from build123d import *

# Parameters (mm, degrees)
SKETCH_1_R      = 1.4
EXTRUDE_1_DEPTH = 7


with BuildPart() as part:
    # 草图1 → 凸台-拉伸1 (new body)
    with BuildSketch(Plane.XY):
        with BuildLine():
            Line((-42.056135012, 57.617545139), (22.139601015, 67.811046791))
            ThreePointArc((22.139601015, 67.811046791), (31.867424404, 60.749216142), (24.805593755, 51.021392753))
            Line((24.805593755, 51.021392753), (-39.390142272, 40.827891101))
            ThreePointArc((-39.390142272, 40.827891101), (-40.473181997, 40.726394111), (-41.560315394, 40.764045938))
            ThreePointArc((-41.560315394, 40.764045938), (-42.147831339, 41.031589211), (-42.44945072, 41.60236074))
            Line((-42.44945072, 41.60236074), (-44.725061471, 55.933501507))
            ThreePointArc((-44.725061471, 55.933501507), (-44.615083087, 56.569629752), (-44.139340913, 57.006005475))
            ThreePointArc((-44.139340913, 57.006005475), (-43.117343546, 57.378561601), (-42.056135012, 57.617545139))
        make_face()
        with Locations((-30.846871561, 50.790949144)):
            Circle(SKETCH_1_R, mode=Mode.SUBTRACT)
        with Locations((13.596330304, 57.847988749)):
            Circle(SKETCH_1_R, mode=Mode.SUBTRACT)
        with BuildLine():
            Line((6.834080281, 59.305546509), (7.618195793, 54.367412968))
            ThreePointArc((7.618195793, 54.367412968), (5.915048401, 52.021290857), (3.568926289, 53.724438249))
            Line((3.568926289, 53.724438249), (2.784810778, 58.662571789))
            ThreePointArc((2.784810778, 58.662571789), (4.48795817, 61.008693901), (6.834080281, 59.305546509))
        make_face(mode=Mode.SUBTRACT)
        with BuildLine():
            Line((-0.079306676, 58.207784793), (0.704808836, 53.269651252))
            ThreePointArc((0.704808836, 53.269651252), (-0.998338556, 50.923529141), (-3.344460667, 52.626676532))
            Line((-3.344460667, 52.626676532), (-4.128576179, 57.564810073))
            ThreePointArc((-4.128576179, 57.564810073), (-2.425428787, 59.910932184), (-0.079306676, 58.207784793))
        make_face(mode=Mode.SUBTRACT)
        with BuildLine():
            Line((-6.992693633, 57.110023076), (-6.208578121, 52.171889536))
            ThreePointArc((-6.208578121, 52.171889536), (-7.911725513, 49.825767424), (-10.257847624, 51.528914816))
            Line((-10.257847624, 51.528914816), (-11.041963136, 56.467048357))
            ThreePointArc((-11.041963136, 56.467048357), (-9.338815744, 58.813170468), (-6.992693633, 57.110023076))
        make_face(mode=Mode.SUBTRACT)
        with BuildLine():
            Line((-13.906080589, 56.01226136), (-13.121965078, 51.074127819))
            ThreePointArc((-13.121965078, 51.074127819), (-14.82511247, 48.728005708), (-17.171234581, 50.4311531))
            Line((-17.171234581, 50.4311531), (-17.955350093, 55.36928664))
            ThreePointArc((-17.955350093, 55.36928664), (-16.252202701, 57.715408752), (-13.906080589, 56.01226136))
        make_face(mode=Mode.SUBTRACT)
        with BuildLine():
            Line((-20.819467546, 54.914499643), (-20.035352035, 49.976366103))
            ThreePointArc((-20.035352035, 49.976366103), (-21.738499426, 47.630243992), (-24.084621538, 49.333391383))
            Line((-24.084621538, 49.333391383), (-24.868737049, 54.271524924))
            ThreePointArc((-24.868737049, 54.271524924), (-23.165589658, 56.617647035), (-20.819467546, 54.914499643))
        make_face(mode=Mode.SUBTRACT)
    extrude(amount=EXTRUDE_1_DEPTH)


solid = part.part
Design review of the part built by this model. Coordinates are the model's own, in mm. A direction names the side the tool comes from. Give positions to 0.01 mm unless a question says otherwise; leave off trailing zeros. Order: outer loops, then holes, each group sorted by start corner. A loop starts at its lowest first (then second) coordinate and runs counter-clockwise, first axis right, second up. Notation, with made-up numbers: (56, 66.25) - (104, 66.25) arc R21 cw to (104, 81.25) - close; hole circle Ø10 at (79, 37). An arc over 180 degrees is marked (long way). Write item = value, one per line. Start each with the question number.
Q1. We need section B-B on z = 2.5. State how many separate pieces and enclosed holes the cut face has, plus the area to 3 significant figures.
Q2. Clearance check with flat-ended pins moving along their axes: pin 1 Ø3 at (x, z) = (-28, 6) entering from +Y; pin 2 Ø1.5 at (x, z) = (-14.5, 3.5) entering from +Y; pin 3 Ø3 at (x, z) = (-3, 1.5) entering from +Y. State where each tip first meets the part, or that it passes through.
Q3. Tool access review of faces 4 (the face through (-16.297, 57.708, 3.451)), 5 (the face through (-6.843, 45.996, 3.451)): name each direction out of +Z, -Z, +X, -X, +Y, -Y from which nothing blocks a thin tool from reaching the whole face with its end or side.
Q4. Mouldability with a two-part tool opening along Y and no side actions: class faces 1 (the face through (-43.132, 57.374, 3.451)), 2 (the face through (-13.52, 53.58, 3.45)), 3 (the face through (-6, 55, 7)) as released by +Y, released by -Y, zero draft, split by the parting line, or undercut.
Q5. We need section C-C on x = 6. State the section outline as (y, z) points.
Q6. We need section A-A on x = -15.5. State the section outline as (y, z) points, plus the area to 3 significant figures.
Q7. To check wall thickness, follow L1, parallel to X at y = 55.25, z = 1.25; L2, parallel to X at y = 54.25, z = 3.5; L3, parallel to Y at x = -3, z = 5.75. State the ranges of each line that lie inside material, in increasing order. Write a range as from..to.
Working result:
q1.separate_pieces = 1
q1.enclosed_holes = 7
q1.area = 1,090 mm²
q2.pin_1 = 60.09
q2.pin_2 = 62.11
q2.pin_3 = 64.06
q3.face_4 = +Z, -Z
q3.face_5 = +Z, -Z, +X, -Y
q4.face_1 = released by +Y
q4.face_2 = undercut
q4.face_3 = zero draft
q5.outline = (48.04, 0) - (52.04, 0) - (52.04, 7) - (48.04, 7) - close; (60.65, 0) - (65.25, 0) - (65.25, 7) - (60.65, 7) - close
q6.outline = (44.62, 0) - (48.73, 0) - (48.73, 7) - (44.62, 7) - close; (57.7, 0) - (61.83, 0) - (61.83, 7) - (57.7, 7) - close
q6.area = 57.8 mm²
q7.L1 = -44.62..-24.79, -20.9..-17.94, -13.79..-10.85, -6.7..-3.76, 0.39..3.33, 7.48..30.88
q7.L2 = -44.46..-24.87, -20.71..-17.78, -13.63..-10.69, -6.54..-3.6, 0.55..3.49, 7.63..30.22
q7.L3 = 46.61..51.77, 59.73..63.82
